from build123d import *

# Parameters (mm, degrees)
F2_W     = 44.45
F2_H     = 12.7
F3_DEPTH = 12.7
F4_R     = 0.381
F5_DEPTH = 12.701
F7_DEPTH = 12.7


with BuildPart() as f3:
    # F2 (on face) → F3 (new body)
    with BuildSketch(Plane.XY):
        with Locations((-0.8636, -0.9906)):
            Rectangle(F2_W, F2_H)
    extrude(amount=F3_DEPTH)

    # F4 (on face) → F5 (cut, through all)
    with BuildSketch(Plane.XY.offset(12.7)):
        with Locations((-18.20926, -5.9944)):
            Circle(F4_R)
        with Locations((-15.66926, -5.9944)):
            Circle(F4_R)
        with Locations((-13.12926, -5.9944)):
            Circle(F4_R)
        with Locations((-14.3764, -2.1971)):
            Circle(F4_R)
        with Locations((-15.6464, -2.1971)):
            Circle(F4_R)
        with Locations((-15.6464, -0.9271)):
            Circle(F4_R)
        with Locations((-14.3764, -0.9271)):
            Circle(F4_R)
        with Locations((-14.3764, 0.3429)):
            Circle(F4_R)
        with Locations((-15.6464, 0.3429)):
            Circle(F4_R)
        with Locations((-4.81076, 0.94742)):
            Circle(F4_R)
        with Locations((5.30352, -3.87604)):
            Circle(F4_R)
        with Locations((5.01904, -2.49936)):
            Circle(F4_R)
        with Locations((6.13918, 1.08712)):
            Circle(F4_R)
        with Locations((5.95884, 3.50774)):
            Circle(F4_R)
        with Locations((8.78586, 3.46964)):
            Circle(F4_R)
        with Locations((18.51914, -0.19304)):
            Circle(F4_R)
        with Locations((16.76273, 3.82016)):
            Circle(F4_R)
        with Locations((14.224, 3.82016)):
            Circle(F4_R)
        with Locations((7.97306, -6.18236)):
            Circle(F4_R)
        with Locations((15.12062, -6.12648)):
            Circle(F4_R)
    extrude(amount=-F5_DEPTH, mode=Mode.SUBTRACT)

    # F6 (on face) → F7 (join, through all)
    with BuildSketch(Plane.XY.offset(12.7)):
        Polygon((-7.2136, -12.4206), (-0.8636, -7.3406), (-5.9436, -7.3406), (-12.2936, -12.4206), align=None)
        Polygon((10.5664, -12.4206), (4.2164, -7.3406), (-0.8636, -7.3406), (5.4864, -12.4206), align=None)
    extrude(amount=-F7_DEPTH)


solid = f3.part
Verification items for the finished model (mm, model axes). A direction names the side the tool comes from. Give positions to 0.01 mm unless a question says otherwise; leave off trailing zeros. Order: outer loops, then holes, each group sorted by start corner. A loop starts at its lowest first (then second) coordinate and runs counter-clockwise, first axis right, second up. Notation, with made-up numbers: M 86.5,-3 L 145.5,-3 A30 ccw 145.5,20 Z; hole C 0.25,24 d7. An arc over 180 degrees is marked long. Use one line per item in the form item = value. Start each with the question number.
Q1. Mould release check, pull along Y, two halves, no side actions. Record for faces 1 (the flat face through (8, -12.421, 6)), 2 (the flat face through (-1, 5.359, 6)), 3 (the flat face through (-9.074, -9.845, 6.439)): +Y half, -Y half, draft (parallel to the pull), parting line (faces both ways), or undercut.
Q2. Section check C-C (x = -1.5). Enter the section's corners in (y, z), then the cut area to 3 significant figures.
Q3. Section check A-A (y = -10.25). Enter the section's corners in (x, z), then the cut area to 3 significant figures.
Q4. Scan lines: line 1 along X through (y, z) = (-1, 11); line 2 along X through (y, z) = (-2.25, 5); line 3 along X through (y, z) = (3.5, 1). Record each from-to range of solid material in increasing order. Write a range as [from, to].
Q5. Section check D-D (x = 11). Enter the section's corners in (y, z), then the cut area to 3 significant figures.
Q6. Section check B-B (z = 11.5). Count the separate pieces of the cut face and the enclosed holes in it, then the cut area to 3 significant figures.
Q7. Access from +Z, -Z, +X, -X, +Y, -Y to the whole of each face (thin tool, end or side, straight path). Record for faces 4 (the flat face through (2.27, -9.85, 6.44)), 5 (the flat face through (-1, -1, 12.7)), 6 (the flat face through (-1, -1, 0)), 7 (the flat face through (-15, -7.341, 6)), 8 (the flat face through (13, -7.341, 6)).
Evaluation:
q1.face_1 = -Y half
q1.face_2 = +Y half
q1.face_3 = undercut
q2.outline = M -7.85,0 L 5.36,0 L 5.36,12.7 L -7.85,12.7 Z
q2.area = 168 mm2
q3.outline = M -9.58,0 L -4.5,0 L -4.5,12.7 L -9.58,12.7 Z; M 2.77,0 L 7.85,0 L 7.85,12.7 L 2.77,12.7 Z
q3.area = 129 mm2
q4.line_1 = [-23.09, -16.02], [-15.27, -14.75], [-14, 21.36]
q4.line_2 = [-23.09, -16.02], [-15.27, -14.75], [-14, 4.73], [5.31, 21.36]
q4.line_3 = [-23.09, 5.58], [6.34, 8.41], [9.17, 14.02], [14.43, 16.56], [16.97, 21.36]
q5.outline = M -7.34,0 L 5.36,0 L 5.36,12.7 L -7.34,12.7 Z
q5.area = 161 mm2
q6.separate_pieces = 1
q6.enclosed_holes = 20
q6.area = 607 mm2
q7.face_4 = +Z, -Z, -Y
q7.face_5 = +Z, +X, -X, +Y, -Y
q7.face_6 = -Z, +X, -X, +Y, -Y
q7.face_7 = +Z, -Z, -X
q7.face_8 = +Z, -Z, +X
